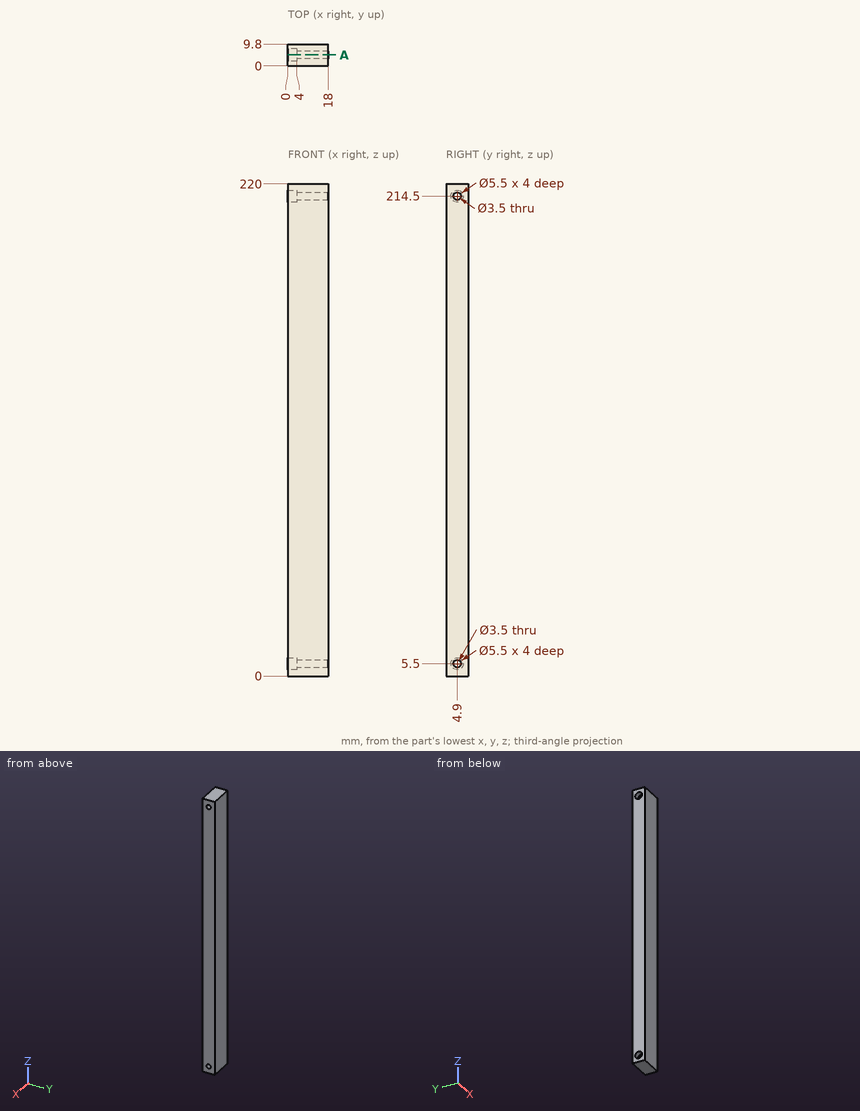
For this review, use the dimensioned drawing (mm, ordinates from the lowest corner) and the shaded views. Give positions to 0.01 mm unless a question says otherwise; leave off trailing zeros. Write each loop counter-clockwise with the first axis right and the second up, starting at its lowest first coordinate (ties: lowest second). Pieces come first, ordered by that corner, then holes. Notation, with made-up numbers: M 82.5,-10 L 116.5,-10 A15 cw 116.5,4 Z; hole C 34,-34 d1. An arc over 180 degrees is marked long. Answer as a JSON object with one key per item and string values. Group by question number.
1) Clearance check with a flat-ended pin moving along its axis: pin 1 Ø1.6 at (y, z) = (4.5, 213.5) entering from -X. State where the tip first meets the part, or that it passes through.
2) We need section A-A (y = 4.9). Give the boundary of the cut face in (x, z).
3) For line 1 along Z through (x, y) = (7, 4.5); line 2 along Z through (x, y) = (3.25, 3.5); line 3 along Y through (x, z) = (7.75, 214.5), list the stretches that pass through material, from the lowest coordinate up.
Answer key:
{
 "1": {"pin 1": "stops at x = 4"},
 "2": {"outline": "M 0,0 L 18,0 L 18,3.75 L 4,3.75 L 4,2.75 L 0,2.75 Z; M 0,8.25 L 4,8.25 L 4,7.25 L 18,7.25 L 18,212.75 L 4,212.75 L 4,211.75 L 0,211.75 Z; M 0,217.25 L 4,217.25 L 4,216.25 L 18,216.25 L 18,220 L 0,220 Z"},
 "3": {"line 1": "z = 0 to 3.8, 7.2 to 212.8, 216.2 to 220", "line 2": "z = 0 to 3.13, 7.87 to 212.13, 216.87 to 220", "line 3": "y = 0 to 3.15, 6.65 to 9.8"}
}
